Can you work these out from the drawing? Everything is in mm from the part's minimum corner. Give positions to 0.01 mm unless a question says otherwise; leave off trailing zeros. Write each loop counter-clockwise with the first axis right and the second up, starting at its lowest first coordinate (ties: lowest second). Pieces come first, ordered by that corner, then holes. Notation, with made-up numbers: (21.25, 29.25) -> (78.25, 29.25) arc R19 ccw to (78.25, 65.25) -> close; hole circle Ø7 at (-38.5, 24). An arc over 180 degrees is marked (long way). Return JSON: item names as keys, results as strings.
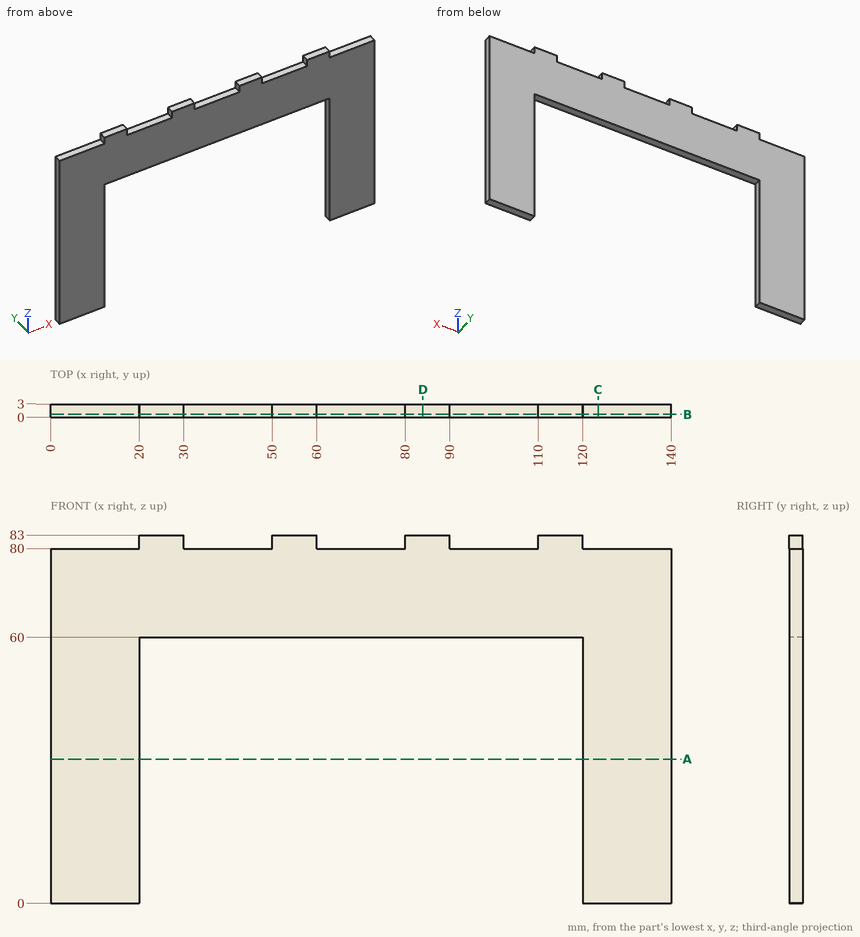
1. Suppose I cut it at C-C, the plane x = 123.5. List the corners of the cut face in (y, z) for me.
Taken from the geometry:
{"outline": "(0, 0) -> (3, 0) -> (3, 80) -> (0, 80) -> close"}
2. Suppose I cut it at B-B, the plane y = 0.65. List the corners of the cut face in (x, z) for me, and give its area (3 significant figures).
Taken from the geometry:
{"outline": "(0, 0) -> (20, 0) -> (20, 60) -> (120, 60) -> (120, 0) -> (140, 0) -> (140, 80) -> (120, 80) -> (120, 83) -> (110, 83) -> (110, 80) -> (90, 80) -> (90, 83) -> (80, 83) -> (80, 80) -> (60, 80) -> (60, 83) -> (50, 83) -> (50, 80) -> (30, 80) -> (30, 83) -> (20, 83) -> (20, 80) -> (0, 80) -> close", "area": "5,320 mm²"}
3. If I drill on line 1 (X direction, y = 2.7, z = 7); line 2 (Z direction, x = 102.5, y = 0.4); line 3 (Z direction, x = 117, y = 1.6), over which ranges is the centre line in solid material (lowest first)? Write a range as [from, to].
Taken from the geometry:
{"line 1": "x = [0, 20], [120, 140]", "line 2": "z = [60, 80]", "line 3": "z = [60, 83]"}
4. Suppose I cut it at D-D, the plane x = 84. List the corners of the cut face in (y, z) for me.
Taken from the geometry:
{"outline": "(0, 60) -> (3, 60) -> (3, 83) -> (0, 83) -> close"}
5. For pin 1 Ø1.5 at (y, z) = (2, 81) entering from +X; pin 2 Ø0.9 at (y, z) = (2, 81.5) entering from -X, each with a flat end and sliding along its axis, tell me the tip position at first contact or that it passes through.
Taken from the geometry:
{"pin 1": "stops at x = 120", "pin 2": "stops at x = 20"}
6. Suppose I cut it at A-A, the plane z = 32.5. List the corners of the cut face in (x, y) for me, and give its area (3 significant figures).
Taken from the geometry:
{"outline": "(0, 0) -> (20, 0) -> (20, 3) -> (0, 3) -> close; (120, 0) -> (140, 0) -> (140, 3) -> (120, 3) -> close", "area": "120 mm²"}
